```python
from build123d import *

# Parameters (mm, degrees)
BOSS_EXTRUDE1_DEPTH = 10
CUT_EXTRUDE1_REACH  = 22
SKETCH2_R           = 1.55
CUT_EXTRUDE2_REACH  = 17
SKETCH3_R           = 1.65


with BuildPart() as part:
    # Sketch1 → Boss-Extrude1 (new body)
    with BuildSketch(Plane(origin=(0, 0, 0), x_dir=(1, 0, 0), z_dir=(0, 1, 0))):
        Polygon((0, 0), (17, 0), (17, -12), (20, -12), (20, 3), (0, 3), align=None)
    extrude(amount=BOSS_EXTRUDE1_DEPTH)

    # Sketch2 → Cut-Extrude1 (cut, up to next)
    with BuildSketch(Plane(origin=(20, 0, 0), x_dir=(0, 0, -1), z_dir=(1, 0, 0)), mode=Mode.PRIVATE) as cut_extrude1_sk1:
        with Locations((-6, 5)):
            Circle(SKETCH2_R)
    cut_extrude1_tool1 = extrude(cut_extrude1_sk1.sketch, amount=-CUT_EXTRUDE1_REACH, mode=Mode.PRIVATE) & part.part
    add(cut_extrude1_tool1.solids().sort_by_distance((20, 5, 6))[0], mode=Mode.SUBTRACT)

    # Sketch3 → Cut-Extrude2 (cut, up to next)
    with BuildSketch(Plane(origin=(0, 0, -3), x_dir=(-1, 0, 0), z_dir=(0, 0, -1)), mode=Mode.PRIVATE) as cut_extrude2_sk1:
        with Locations((-9.4, 5)):
            Circle(SKETCH3_R)
    cut_extrude2_tool1 = extrude(cut_extrude2_sk1.sketch, amount=-CUT_EXTRUDE2_REACH, mode=Mode.PRIVATE) & part.part
    add(cut_extrude2_tool1.solids().sort_by_distance((9.4, 5, -3))[0], mode=Mode.SUBTRACT)


solid = part.part
```
Model file for the job. Use its own axes, mm. A direction names the side the tool comes from. Coordinates: 2 decimals unless noted, no trailing zeros. Loops run counter-clockwise (first coordinate to the right, second up) from the corner with the lowest first, then second, coordinate; pieces in that order, holes last. Notation, with made-up numbers: (55, 55) - (87, 55) arc R18 ccw to (87, 85) - close; hole circle Ø10 at (81.25, 34). An arc over 180 degrees is marked (long way). Answer as a JSON object with one key per item and string values. Group by question number.
(1) Tool access for faces 4 (the face through (13, 0, -2)), 5 (the face through (6, 5, 0)): list every direction of +Z, -Z, +X, -X, +Y, -Y with a clear straight run to the whole face (end or side of a thin tool).
(2) Flat gauge pin, fed straight in: pin 1 (4 mm diameter, centred on x = 10, y = 9, fed in from +Z). Where does the tip first touch, or does it go through?
(3) Two-plate mould, pull along Z, no slides. Class faces 1 (the face through (17, 3.8, 4.6)), 2 (the face through (12, 5, -3)), 3 (the face through (18.52, 5.07, 7.55)): released by +Z, released by -Z, zero draft, split by the parting line, or undercut.
(4) Cut at D-D (z = 1.75). Give the cut face in (x, y).
(5) Cut at B-B (y = 5). Give the cut face in (x, z), then the cut area to 3 significant figures.
(6) Cut at A-A (z = 6). Give the cut face in (x, y).
(7) Cut at C-C (x = 8). Give the cut face in (y, z).
(8) Probe line 1 along Y through (x, z) = (19.3, 6); line 2 along Y through (x, z) = (9.4, -0.85); line 3 along Z through (x, y) = (7.75, 4). List the from-to ranges inside material, lowest first.
Geometry says:
{
 "1": {"face 4": "+Z, -Z, +X, -X, -Y", "face 5": "+Z, -X, +Y, -Y"},
 "2": {"pin 1": "stops at z = 0"},
 "3": {"face 1": "zero draft", "face 2": "released by -Z", "face 3": "undercut"},
 "4": {"outline": "(17, 0) - (20, 0) - (20, 10) - (17, 10) - close"},
 "5": {"outline": "(0, -3) - (7.75, -3) - (7.75, 0) - (0, 0) - close; (11.05, -3) - (20, -3) - (20, 4.45) - (17, 4.45) - (17, 0) - (11.05, 0) - close; (17, 7.55) - (20, 7.55) - (20, 12) - (17, 12) - close", "area": "76.8 mm^2"},
 "6": {"outline": "(17, 0) - (20, 0) - (20, 3.45) - (17, 3.45) - close; (17, 6.55) - (20, 6.55) - (20, 10) - (17, 10) - close"},
 "7": {"outline": "(0, -3) - (4.13, -3) - (4.13, 0) - (0, 0) - close; (5.87, -3) - (10, -3) - (10, 0) - (5.87, 0) - close"},
 "8": {"line 1": "y = 0 to 3.45, 6.55 to 10", "line 2": "y = 0 to 3.35, 6.65 to 10", "line 3": "z = -3 to 0"}
}
